CAD build for the part. Positions are in the model's coordinates, mm. Face numbers are marked on the shaded views. A direction names the side the tool comes from. Give positions to 0.01 mm unless a question says otherwise; leave off trailing zeros. Order: outer loops, then holes, each group sorted by start corner. A loop starts at its lowest first (then second) coordinate and runs counter-clockwise, first axis right, second up. Notation, with made-up numbers: (4.5, 71.5) -> (16.5, 71.5) arc R27 cw to (16.5, 110.5) -> close; hole circle Ø4 at (74.5, -26.75). An arc over 180 degrees is marked (long way). Answer as CSV lines item,"result".
```python
from build123d import *

# Parameters (mm, degrees)
SKETCH1_R           = 1
BOSS_EXTRUDE1_DEPTH = 2
SKETCH2_R           = 2
CUT_EXTRUDE1_DEPTH  = 1
BOSS_EXTRUDE2_DEPTH = 2
BOSS_EXTRUDE3_DEPTH = 1


with BuildPart() as part:
    # Sketch1 → Boss-Extrude1 (new body)
    with BuildSketch(Plane.XY):
        with BuildLine():
            Line((3, 0), (3, 3))
            Line((3, 3), (0, 3))
            ThreePointArc((0, 3), (-3, 0), (0, -3))
            ThreePointArc((0, -3), (2.121320344, -2.121320344), (3, 0))
        make_face()
        Circle(SKETCH1_R, mode=Mode.SUBTRACT)
    extrude(amount=BOSS_EXTRUDE1_DEPTH)

    # Sketch2 → Cut-Extrude1 (cut)
    with BuildSketch(Plane.XY.offset(2)):
        Circle(SKETCH2_R)
    extrude(amount=-CUT_EXTRUDE1_DEPTH, mode=Mode.SUBTRACT)

    # Sketch3 → Boss-Extrude2 (add)
    with BuildSketch(Plane.XY.offset(2)):
        with BuildLine():
            Line((0, -2), (0, -3))
            ThreePointArc((0, -3), (2.121320344, -2.121320344), (3, 0))
            Line((3, 0), (2, 0))
            Line((2, 0), (1, 0))
            ThreePointArc((1, 0), (0.707106781, -0.707106781), (0, -1))
            Line((0, -1), (0, -2))
        make_face()
    extrude(amount=BOSS_EXTRUDE2_DEPTH)

    # Sketch4 → Boss-Extrude3 (add)
    with BuildSketch(Plane.XY.offset(2)):
        with BuildLine():
            Line((-3, 0), (-2, 0))
            Line((-2, 0), (-1, 0))
            ThreePointArc((-1, 0), (-0.707106781, -0.707106781), (0, -1))
            Line((0, -1), (0, -2))
            Line((0, -2), (0, -3))
            ThreePointArc((0, -3), (-2.121320344, -2.121320344), (-3, 0))
        make_face()
    extrude(amount=BOSS_EXTRUDE3_DEPTH)


solid = part.part
```
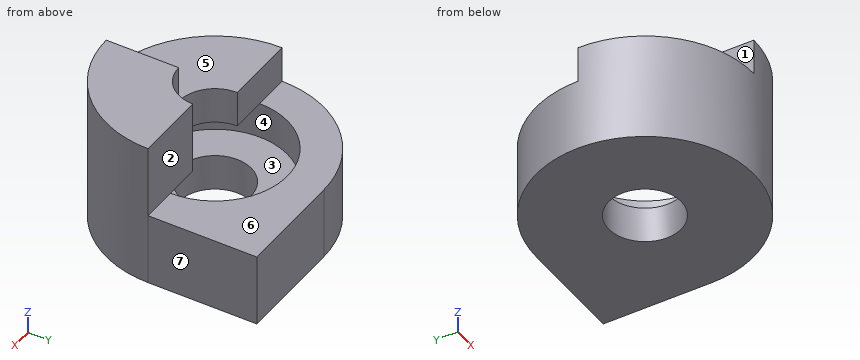
1) Pin check, flat tips, straight feed: P1, Ø2, axis at x = -1, y = -0.5, coming from the +Z side; P2, Ø2.5, axis at x = 0, y = 0, coming from the +Z side; P3, Ø0.5, axis at x = -1.5, z = 2.5, coming from the +Y side; P4, Ø1.5, axis at x = 0.5, y = 1, coming from the +Z side. Stop position of each tip, or through.
Data:
P1,"stops at z = 3"
P2,"stops at z = 4"
P3,"stops at y = 0"
P4,"stops at z = 1"
2) Band-saw the part on B-B, the plane x = 0.45. Write the cut outline in (y, z), then the cut area to 3 significant figures.
Data:
outline,"(-2.97, 0) -> (-0.89, 0) -> (-0.89, 1) -> (-1.95, 1) -> (-1.95, 2) -> (-0.89, 2) -> (-0.89, 4) -> (-2.97, 4) -> close; (0.89, 0) -> (3, 0) -> (3, 2) -> (1.95, 2) -> (1.95, 1) -> (0.89, 1) -> close"
area,"10.4 mm2"
3) Band-saw the part on D-D, the plane z = 1.55. Write the cut outline in (x, y), then the cut area to 3 significant figures.
Data:
outline,"(0, 3) arc R3 ccw (long way) to (3, 0) -> (3, 3) -> close; hole circle Ø4 at (0, 0)"
area,"17.6 mm2"
4) Wall check: line 1 along Z through (x, y) = (0.4, -1.2); line 2 along Y through (x, z) = (0, 1.3); line 3 along Y through (x, z) = (0, 0.45). Give the ranges that are in metal, low to high. Write a range as [from, to].
Data:
line 1,"z = [0, 1], [2, 4]"
line 2,"y = [-3, -2], [2, 3]"
line 3,"y = [-3, -1], [1, 3]"
5) Band-saw the part on A-A, the plane y = -0.45. Write the cut outline in (x, z), then the cut area to 3 significant figures.
Data:
outline,"(-2.97, 0) -> (-0.89, 0) -> (-0.89, 1) -> (-1.95, 1) -> (-1.95, 2) -> (-0.89, 2) -> (-0.89, 3) -> (-2.97, 3) -> close; (0.89, 0) -> (2.97, 0) -> (2.97, 4) -> (0.89, 4) -> (0.89, 2) -> (1.95, 2) -> (1.95, 1) -> (0.89, 1) -> close"
area,"12.4 mm2"
6) Which spindle directions (+Z, -Z, +X, -X, +Y, -Y) get a long thin tool onto all of the face, cutting with end or side? Do the marked faces 5, 6 and 7. Say none if no direction does.
Data:
face 5,"+Z, -X, +Y, -Y"
face 6,"+Z, +X, -X, +Y"
face 7,"+Z, -Z, +X, +Y, -Y"
7) Pull direction X, two halves, no side cores. Call the marked faces 1, 2, 3 and 4: pulls with the +X half, pulls with the -X half, needs draft (parallel to the pull), parting line crosses it, or undercut.
Data:
face 1,"pulls with the -X half"
face 2,"needs draft"
face 3,"undercut"
face 4,"undercut"
8) Band-saw the part on C-C, the plane y = -1.25. Write the cut outline in (x, z), then the cut area to 3 significant figures.
Data:
outline,"(-2.73, 0) -> (2.73, 0) -> (2.73, 4) -> (0, 4) -> (0, 3) -> (-2.73, 3) -> close; hole (-1.56, 1) -> (1.56, 1) -> (1.56, 2) -> (-1.56, 2) -> close"
area,"16.0 mm2"
